Geometry: final body of the model. Coordinates: model frame, mm. Coordinates: 2 decimals unless noted, no trailing zeros. Order: outer loops, then holes, each group sorted by start corner. A loop starts at its lowest first (then second) coordinate and runs counter-clockwise, first axis right, second up. Notation, with made-up numbers: M 52,78 L 65,78 A26 ccw 65,92 Z; hole C 18.5,27 d5. An arc over 180 degrees is marked long. Write item = value, one per line.
from build123d import *

# Parameters (mm, degrees)
SWEEP1_PROFILE_R = 6.35


with BuildPart() as part:
    # Sweep1: sweep along a path in Sketch2
    with BuildLine(Plane.XY) as sweep1_path:
        Line((-121.321774851, 25.344617349), (-79.496231466, -31.161414773))
        Line((-79.496231466, -31.161414773), (11.079614142, -33.931318309))
        Line((11.079614142, -33.931318309), (64.538752375, -9.556167197))
        Line((64.538752375, -9.556167197), (123.260707326, -18.419858511))
        Line((123.260707326, -18.419858511), (182.813633337, 2.631408359))
        Line((182.813633337, 2.631408359), (206.911794096, -39.194135026))
    # Sweep1 profile (on start of the path) → Sweep1 (sweep)
    with BuildSketch(Plane(origin=(-121.321774851, 25.344617349, 0), x_dir=(-0.8037665341662223, -0.5949448365642138, 0), z_dir=(0.5949448365642138, -0.8037665341662223, 0))):
        Circle(SWEEP1_PROFILE_R)
    sweep(path=sweep1_path.line, transition=Transition.RIGHT)


solid = part.part
1) Section A-A, the plane z = 2.75. Return loops of the section in (x, y).
Numbers:
outline = M -125.92,21.94 L -82.45,-36.8 L 12.24,-39.69 L 65.37,-15.47 L 123.82,-24.29 L 180.23,-4.35 L 201.95,-42.05 L 211.87,-36.34 L 185.4,9.61 L 122.7,-12.55 L 63.71,-3.64 L 9.92,-28.17 L -76.55,-25.53 L -116.72,28.75 Z
2) Line query: L1, parallel to X at y = -36.5, z = -1.5; L2, parallel to Y at x = -21, z = -2.25; L3, parallel to Y at x = 125.5, z = 2.75. Output: solid intervals per line, ascending.
Numbers:
L1 = -83.22 to 20.32, 198.24 to 211.59
L2 = -38.89 to -27.01
L3 = -23.7 to -11.56
3) Mould query, pull axis X, two halves, no side actions, for faces 1 (the face through (93.28, -20.02, -1.91)), 2 (the face through (153.128, -1.134, -0.279)), 3 (the face through (-121.25, 25.4, -0.09)), 4 (the face through (206.99, -39.15, -0.09)). Classes: pulls with the +X half, pulls with the -X half, needs draft (parallel to the pull), parting line crosses it, or undercut.
Numbers:
face_1 = undercut
face_2 = undercut
face_3 = pulls with the -X half
face_4 = pulls with the +X half
4) Pin query (flat end, axial travel): pin 1 (3 mm diameter, centred on y = -30, z = 2, fed in from -X); pin 2 (6 mm diameter, centred on y = -34, z = -3.5, fed in from -X); pin 3 (4 mm diameter, centred on y = -5.5, z = -1, fed in from -X). Return the tip coordinate at first contact, or that it passes through.
Numbers:
pin_1 = -89.08
pin_2 = -86.82
pin_3 = -107.81
